Model file for the job. Use its own axes, mm. A direction names the side the tool comes from. Round coordinates to 2 decimals unless told otherwise and drop trailing zeros. Loops run counter-clockwise (first coordinate to the right, second up) from the corner with the lowest first, then second, coordinate; pieces in that order, holes last.
from build123d import *

# Parameters (mm, degrees)
SKETCH1_R           = 2.5
BOSS_EXTRUDE1_DEPTH = 120


with BuildPart() as part:
    # Sketch1 → Boss-Extrude1 (new body)
    with BuildSketch(Plane.XY):
        with BuildLine():
            Line((-7.427382464, 2.155691805), (-5.727382464, 2.155691805))
            ThreePointArc((-5.727382464, 2.155691805), (-5.621316447, 2.199625788), (-5.577382464, 2.305691805))
            Line((-5.577382464, 2.305691805), (-5.577382464, 5.741876319))
            ThreePointArc((-5.577382464, 5.741876319), (-5.485183419, 5.880292537), (-5.321928469, 5.848550846))
            Line((-5.321928469, 5.848550846), (-1.531086168, 2.101082027))
            Line((-1.531086168, 2.101082027), (-1.531086168, -3.789698417))
            Line((-1.531086168, -3.789698417), (-5.321928469, -7.537167236))
            ThreePointArc((-5.321928469, -7.537167236), (-5.485183419, -7.568908927), (-5.577382464, -7.430492708))
            Line((-5.577382464, -7.430492708), (-5.577382464, -3.994308195))
            ThreePointArc((-5.577382464, -3.994308195), (-5.621316447, -3.888242178), (-5.727382464, -3.844308195))
            Line((-5.727382464, -3.844308195), (-7.427382464, -3.844308195))
            ThreePointArc((-7.427382464, -3.844308195), (-7.533448481, -3.888242178), (-7.577382464, -3.994308195))
            Line((-7.577382464, -3.994308195), (-7.577382464, -10.494308195))
            ThreePointArc((-7.577382464, -10.494308195), (-7.474869837, -10.741795568), (-7.227382464, -10.844308195))
            Line((-7.227382464, -10.844308195), (-0.727382464, -10.844308195))
            ThreePointArc((-0.727382464, -10.844308195), (-0.621316447, -10.800374212), (-0.577382464, -10.694308195))
            Line((-0.577382464, -10.694308195), (-0.577382464, -8.994308195))
            ThreePointArc((-0.577382464, -8.994308195), (-0.621316447, -8.888242178), (-0.727382464, -8.844308195))
            Line((-0.727382464, -8.844308195), (-4.145467261, -8.844308195))
            ThreePointArc((-4.145467261, -8.844308195), (-4.284213755, -8.751311795), (-4.250921257, -8.587633667))
            Line((-4.250921257, -8.587633667), (-0.464270258, -4.844308195))
            Line((-0.464270258, -4.844308195), (5.402097922, -4.844308195))
            Line((5.402097922, -4.844308195), (9.188748921, -8.587633667))
            ThreePointArc((9.188748921, -8.587633667), (9.22204142, -8.751311795), (9.083294926, -8.844308195))
            Line((9.083294926, -8.844308195), (5.665210129, -8.844308195))
            ThreePointArc((5.665210129, -8.844308195), (5.559144111, -8.888242178), (5.515210129, -8.994308195))
            Line((5.515210129, -8.994308195), (5.515210129, -10.694308195))
            ThreePointArc((5.515210129, -10.694308195), (5.559144111, -10.800374212), (5.665210129, -10.844308195))
            Line((5.665210129, -10.844308195), (12.165210129, -10.844308195))
            ThreePointArc((12.165210129, -10.844308195), (12.412697502, -10.741795568), (12.515210129, -10.494308195))
            Line((12.515210129, -10.494308195), (12.515210129, -3.994308195))
            ThreePointArc((12.515210129, -3.994308195), (12.471276146, -3.888242178), (12.365210129, -3.844308195))
            Line((12.365210129, -3.844308195), (10.665210129, -3.844308195))
            ThreePointArc((10.665210129, -3.844308195), (10.559144111, -3.888242178), (10.515210129, -3.994308195))
            Line((10.515210129, -3.994308195), (10.515210129, -7.430492708))
            ThreePointArc((10.515210129, -7.430492708), (10.423011083, -7.568908927), (10.259756133, -7.537167236))
            Line((10.259756133, -7.537167236), (6.468913832, -3.789698417))
            Line((6.468913832, -3.789698417), (6.468913832, 2.101082027))
            Line((6.468913832, 2.101082027), (10.259756133, 5.848550846))
            ThreePointArc((10.259756133, 5.848550846), (10.423011083, 5.880292537), (10.515210129, 5.741876319))
            Line((10.515210129, 5.741876319), (10.515210129, 2.305691805))
            ThreePointArc((10.515210129, 2.305691805), (10.559144111, 2.199625788), (10.665210129, 2.155691805))
            Line((10.665210129, 2.155691805), (12.365210129, 2.155691805))
            ThreePointArc((12.365210129, 2.155691805), (12.471276146, 2.199625788), (12.515210129, 2.305691805))
            Line((12.515210129, 2.305691805), (12.515210129, 8.805691805))
            ThreePointArc((12.515210129, 8.805691805), (12.412697502, 9.053179179), (12.165210129, 9.155691805))
            Line((12.165210129, 9.155691805), (5.665210129, 9.155691805))
            ThreePointArc((5.665210129, 9.155691805), (5.559144111, 9.111757822), (5.515210129, 9.005691805))
            Line((5.515210129, 9.005691805), (5.515210129, 7.305691805))
            ThreePointArc((5.515210129, 7.305691805), (5.559144111, 7.199625788), (5.665210129, 7.155691805))
            Line((5.665210129, 7.155691805), (9.083294926, 7.155691805))
            ThreePointArc((9.083294926, 7.155691805), (9.22204142, 7.062695405), (9.188748921, 6.899017277))
            Line((9.188748921, 6.899017277), (5.402097922, 3.155691805))
            Line((5.402097922, 3.155691805), (-0.464270258, 3.155691805))
            Line((-0.464270258, 3.155691805), (-4.250921257, 6.899017277))
            ThreePointArc((-4.250921257, 6.899017277), (-4.284213755, 7.062695405), (-4.145467261, 7.155691805))
            Line((-4.145467261, 7.155691805), (-0.727382464, 7.155691805))
            ThreePointArc((-0.727382464, 7.155691805), (-0.621316447, 7.199625788), (-0.577382464, 7.305691805))
            Line((-0.577382464, 7.305691805), (-0.577382464, 9.005691805))
            ThreePointArc((-0.577382464, 9.005691805), (-0.621316447, 9.111757822), (-0.727382464, 9.155691805))
            Line((-0.727382464, 9.155691805), (-7.227382464, 9.155691805))
            ThreePointArc((-7.227382464, 9.155691805), (-7.474869837, 9.053179179), (-7.577382464, 8.805691805))
            Line((-7.577382464, 8.805691805), (-7.577382464, 2.305691805))
            ThreePointArc((-7.577382464, 2.305691805), (-7.533448481, 2.199625788), (-7.427382464, 2.155691805))
        make_face()
        with Locations((2.468913832, -0.844308195)):
            Circle(SKETCH1_R, mode=Mode.SUBTRACT)
    extrude(amount=BOSS_EXTRUDE1_DEPTH)


solid = part.part
Q1. Tool access for faces 4 (the face through (-1.531, -1, 59)), 5 (the face through (8.4, -5.7, 59.2)), 6 (the face through (3, 3.156, 59)), 7 (the face through (6.469, -1, 59)): list every direction of +Z, -Z, +X, -X, +Y, -Y with a clear straight run to the whole face (end or side of a thin tool).
Q2. Pull direction Y, two halves, no side cores. Call faces 1 (the face through (-5.577, 4, 59)), 2 (the face through (2, -4.844, 59)), 3 (the face through (9, 9.156, 59)): pulls with the +Y half, pulls with the -Y half, needs draft (parallel to the pull), parting line crosses it, or undercut.
Q3. Probe line 1 (X direction, y = 8.25, z = 45); line 2 (Y direction, x = 2.25, z = 57); line 3 (Y direction, x = -3, z = 62). List the from-to ranges inside material, lowest first.
Q4. Slice it at A-A on x = 3.25. Give the cut face in (y, z), plus the area to 3 significant figures.
Q5. Slice it at B-B on y = 0.5. Give the cut face in (x, z), plus the area to 3 significant figures.
Q6. Flat gauge pin, fed straight in: P1, Ø1.8, axis at x = 2.5, z = 66.5, coming from the +Y side. Where does the tip first touch, or does it go through?
Reply:
1. face 4: +Z, -Z, -X
1. face 5: +Z, -Z
1. face 6: +Z, -Z, +Y
1. face 7: +Z, -Z, +X
2. face 1: undercut
2. face 2: pulls with the -Y half
2. face 3: pulls with the +Y half
3. line 1: x = -7.58 to -0.58, 5.52 to 12.52
3. line 2: y = -4.84 to -3.33, 1.65 to 3.16
3. line 3: y = -10.84 to -8.84, -7.35 to -5.24, 3.55 to 5.66, 7.16 to 9.16
4. outline: (-4.84, 0) - (-3.22, 0) - (-3.22, 120) - (-4.84, 120) - close; (1.53, 0) - (3.16, 0) - (3.16, 120) - (1.53, 120) - close
4. area: 390 mm2
5. outline: (-1.53, 0) - (0.36, 0) - (0.36, 120) - (-1.53, 120) - close; (4.58, 0) - (6.47, 0) - (6.47, 120) - (4.58, 120) - close
5. area: 454 mm2
6. P1: stops at y = 3.16
